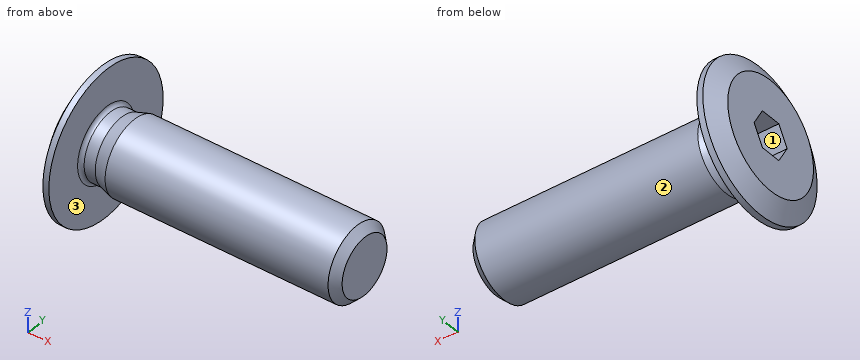
Autodesk Inventor part; units mm, degrees
ref_plane "YZ Plane" through (0, 0, 0) normal (1, 0, 0) x (0, 1, 0)
ref_plane "XZ Plane" through (0, 0, 0) normal (0, 1, 0) x (-1, 0, 0)
ref_plane "XY Plane" through (0, 0, 0) normal (0, 0, 1) x (1, 0, 0)
sketch "Sketch_1" plane through (0, 0, 0) normal (0, 0, 1) x (1, 0, 0)
  line L0 (14, 0) -> (-0.9, 0)
  line L1 (-0.9, 0) -> (-0.9, 3)
  line L2 (-0.9, 3) -> (-0.3226, 4)
  line L3 (-0.3226, 4) -> (0, 4)
  line L4 (0, 4) -> (0, 1.9852)
  arc A0 (0, 1.9852) -> (0.2, 1.7853) centre (0.2, 1.9853) ccw
  line L5 (0.2, 1.7853) -> (0.8, 1.7853)
  line L6 (0.8, 1.7853) -> (1.5, 2)
  line L7 (1.5, 2) -> (13.5705, 2)
  line L8 (13.5705, 2) -> (14, 1.5705)
  line L9 (14, 1.5705) -> (14, 0)
  line L10 (14, 0) -> (-0.9, 0)
revolve "Revolution1" add sketch "Sketch_1" angle 360 about axis through (14, 0, 0) along (1, 0, 0)
thread "Thread1"
sketch "Sketch2" plane through (-0.9, 0, 0) normal (-1, 0, 0) x (0, 0, 1)
  point P0 (0, 0)
hole "Hole1" at (-0.9, 0, 0) direction (1, 0, 0) diameter 2 depth 2.5 tip angle 120
sketch "Sketch_3" plane through (-0.9, 0, 0) normal (1, 0, 0) x (0, 0, -1)
  line L0 (-1, -0.5774) -> (0, -1.1547)
  line L1 (0, -1.1547) -> (1, -0.5774)
  line L2 (1, -0.5774) -> (1, 0.5774)
  line L3 (1, 0.5774) -> (0, 1.1547)
  line L4 (0, 1.1547) -> (-1, 0.5774)
  line L5 (-1, 0.5774) -> (-1, -0.5774)
extrude "Extrusion1" cut sketch "Sketch_3" along normal blind 2.5
properties part number "CBSTSR4-14" material "鋼、炭素鋼"
Model file for the job. Use its own axes, mm. Face numbers are marked on the shaded views. Coordinates: 2 decimals unless noted, no trailing zeros. Order: outer loops, then holes, each group sorted by start corner. A loop starts at its lowest first (then second) coordinate and runs counter-clockwise, first axis right, second up. Notation, with made-up numbers: (5.25, -24.5) -> (63.25, -24.5) arc R26 cw to (63.25, -10.5) -> close; hole circle Ø6 at (87.5, 36). An arc over 180 degrees is marked (long way). Answer as a JSON object with one key per item and string values. Group by question number.
1) Flat gauge pin, fed straight in: pin 1 (3 mm diameter, centred on x = 4, y = 1, fed in from +Z). Where does the tip first touch, or does it go through?
2) Drill centre lines: L1, parallel to Y at x = 10, z = 0.25; L2, parallel to X at y = -2, z = 2; L3, parallel to Z at x = 3, y = 0. Where is each one in solid material? Low to high.
3) Pull direction Y, two halves, no side cores. Call the marked faces 1, 2 and 3: +Y half, -Y half, draft (parallel to the pull), parting line (faces both ways), or undercut.
4) Cut at A-A, the plane x = 9.25. Write the cut outline in (y, z).
Check values:
{
 "1": {"pin 1": "stops at z = 2"},
 "2": {"L1": "y = -1.98 to 1.98", "L2": "x = -0.9 to 0", "L3": "z = -2 to 2"},
 "3": {"face 1": "undercut", "face 2": "parting line", "face 3": "draft"},
 "4": {"outline": "circle Ø4 at (0, 0)"}
}
